```python
from build123d import *

# Parameters (mm, degrees)
BOSS_EXTRUDE1_DEPTH = 190.5
SKETCH2_OUTSIDE_W   = 46.489
SKETCH2_OUTSIDE_H   = 47.459
SKETCH2_OUTSIDE_R   = 3.048
CUT_EXTRUDE1_DEPTH  = 19.05


with BuildPart() as part:
    # Sketch1 → Boss-Extrude1 (new body)
    with BuildSketch(Plane(origin=(0, 0, 0), x_dir=(1, 0, 0), z_dir=(0, 1, 0))):
        Polygon((3.310191022, -4.420128359), (3.310191022, -0.762528359), (0.140765019, 1.063061018), (-3.028660983, -0.762528359), (-3.028660983, -4.420128359), (0.140765019, -6.245717737), align=None)
    extrude(amount=BOSS_EXTRUDE1_DEPTH)

    # Sketch2 outside → Cut-Extrude1 (cut)
    with BuildSketch(Plane(origin=(0, 190.5, 0), x_dir=(1, 0, 0), z_dir=(0, 1, 0))):
        with Locations((0.1405, -2.5915)):
            Rectangle(SKETCH2_OUTSIDE_W, SKETCH2_OUTSIDE_H)
        with Locations(Location((0.146339017, -2.591328359, 0), (0, 0, 270))):
            Circle(SKETCH2_OUTSIDE_R, mode=Mode.SUBTRACT)
    cut_extrude1 = extrude(amount=-CUT_EXTRUDE1_DEPTH, mode=Mode.SUBTRACT)

    # Mirror1: Cut-Extrude1 across plane
    add(cut_extrude1.mirror(Plane.ZX.offset(95.25)), mode=Mode.SUBTRACT)


solid = part.part
```
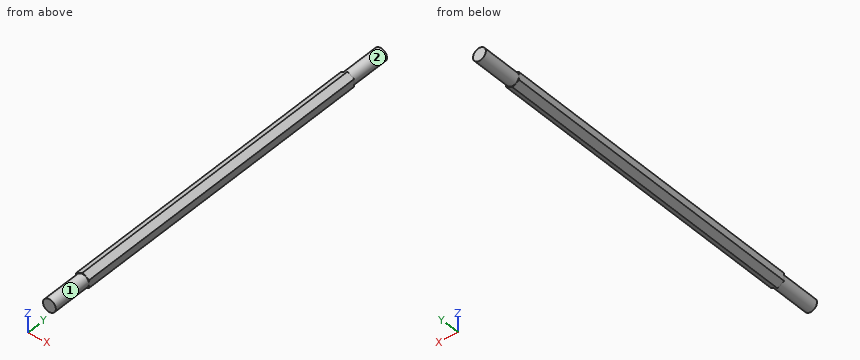
The listing builds one solid part. Answer for the finished solid, in the listing's coordinates (mm). Face numbers are marked on the shaded views. A direction names the side the tool comes from. Round coordinates to 2 decimals unless told otherwise and drop trailing zeros. Order: outer loops, then holes, each group sorted by start corner. A loop starts at its lowest first (then second) coordinate and runs counter-clockwise, first axis right, second up. Notation, with made-up numbers: (44.25, 24) -> (84.25, 24) arc R36 cw to (84.25, 60) -> close; hole circle Ø1 at (72, 39.25). An arc over 180 degrees is marked (long way). Answer as CSV lines item,"result". Start each with the question number.
(1) The part is cut by section B-B (y = 69). Determine the outline of the cut face in (x, z), then the cut area to 3 significant figures.
(2) A tool of negligible diameter and unlimited length cuts with its end or side. For the marked faces 1 and 2, from which of +Z, -Z, +X, -X, +Y, -Y can it reach the whole face along a straight path? Write none if from no direction.
(3) Find the intervals of material crossed by probe 1 along X at (y, z) = (102.5, 4.5); probe 2 along Y at (x, z) = (-0.75, -0.5); probe 3 along Z at (x, y) = (3, 129), in increasing order. Write a range as from..to.
(4) The part is cut by section A-A (x = -1.75). Determine the outline of the cut face in (y, z).
Evaluation:
1,outline,"(-3.03, 0.76) -> (0.14, -1.06) -> (3.31, 0.76) -> (3.31, 4.42) -> (0.14, 6.25) -> (-3.03, 4.42) -> close"
1,area,"34.8 mm²"
2,face 1,"-Y"
2,face 2,"+Y"
3,probe 1,"-2.89..3.17"
3,probe 2,"19.05..171.45"
3,probe 3,"0.58..4.6"
4,outline,"(0, 0.21) -> (19.05, 0.21) -> (19.05, 0.03) -> (171.45, 0.03) -> (171.45, 0.21) -> (190.5, 0.21) -> (190.5, 4.98) -> (171.45, 4.98) -> (171.45, 5.16) -> (19.05, 5.16) -> (19.05, 4.98) -> (0, 4.98) -> close"
